Could you check a few things on this model? Use its own coordinates, in mm. Round coordinates to 2 decimals unless told otherwise and drop trailing zeros. Loops run counter-clockwise (first coordinate to the right, second up) from the corner with the lowest first, then second, coordinate; pieces in that order, holes last. Notation, with made-up numbers: (52.5, 56.25) -> (94.5, 56.25) arc R13 ccw to (94.5, 68.25) -> close; hole circle Ø11 at (16.5, 45.5). An arc over 180 degrees is marked (long way). Write each question's results on one line, items separated by ' | '.
from build123d import *

# Parameters (mm, degrees)
SKETCH1_W           = 70
SKETCH1_H           = 60
SKETCH1_R           = 2.125
SKETCH1_R_2         = 2.5
SKETCH1_R_3         = 1.5
SKETCH1_R_4         = 6
BOSS_EXTRUDE1_DEPTH = 6


with BuildPart() as part:
    # Sketch1 → Boss-Extrude1 (new body)
    with BuildSketch(Plane(origin=(0, 0, 0), x_dir=(1, 0, 0), z_dir=(0, 1, 0))):
        with Locations((0, -5)):
            Rectangle(SKETCH1_W, SKETCH1_H)
        with Locations((-9.450109616, -25)):
            Circle(SKETCH1_R, mode=Mode.SUBTRACT)
        with Locations((-17.450109616, -25)):
            Circle(SKETCH1_R, mode=Mode.SUBTRACT)
        with Locations((-25, -17.5)):
            Circle(SKETCH1_R_2, mode=Mode.SUBTRACT)
        with Locations((25, -17.5)):
            Circle(SKETCH1_R_2, mode=Mode.SUBTRACT)
        with Locations((-16.22, 0)):
            Circle(SKETCH1_R_3, mode=Mode.SUBTRACT)
        Circle(SKETCH1_R_4, mode=Mode.SUBTRACT)
        with Locations((-25, 17.5)):
            Circle(SKETCH1_R_2, mode=Mode.SUBTRACT)
        with Locations((16.22, 0)):
            Circle(SKETCH1_R_3, mode=Mode.SUBTRACT)
        with Locations((25, 17.5)):
            Circle(SKETCH1_R_2, mode=Mode.SUBTRACT)
    extrude(amount=BOSS_EXTRUDE1_DEPTH)


solid = part.part
1) I'm going to push a flat-ended pin straight in: pin 1 (10 mm diameter, centred on x = -26.5, z = -11, fed in from -Y). Where does the tip first touch, or does it pass through?
Model answer:
pin 1: stops at y = 0
2) I want a section at B-B, the plane x = -25. Write out the boundary of the cut face in (y, z), plus the area to 3 significant figures.
Model answer:
outline: (0, -25) -> (6, -25) -> (6, -20) -> (0, -20) -> close; (0, -15) -> (6, -15) -> (6, 15) -> (0, 15) -> close; (0, 20) -> (6, 20) -> (6, 35) -> (0, 35) -> close | area: 300 mm2
3) I want a section at C-C, the plane z = 0. Write out the boundary of the cut face in (x, y), plus the area to 3 significant figures.
Model answer:
outline: (-35, 0) -> (-17.72, 0) -> (-17.72, 6) -> (-35, 6) -> close; (-14.72, 0) -> (-6, 0) -> (-6, 6) -> (-14.72, 6) -> close; (6, 0) -> (14.72, 0) -> (14.72, 6) -> (6, 6) -> close; (17.72, 0) -> (35, 0) -> (35, 6) -> (17.72, 6) -> close | area: 312 mm2
4) I want a section at A-A, the plane z = 19. Write out the boundary of the cut face in (x, y).
Model answer:
outline: (-35, 0) -> (-27, 0) -> (-27, 6) -> (-35, 6) -> close; (-23, 0) -> (23, 0) -> (23, 6) -> (-23, 6) -> close; (27, 0) -> (35, 0) -> (35, 6) -> (27, 6) -> close
5) If we mould it in two halves opening along X, with no side actions, what happens to faces 1 (the flat face through (7, 6, 5)), 2 (the flat face through (-35, 3, 5)), 3 (the cylindrical face through (-6, 3, 0))? For each: released by +X, released by -X, zero draft, split by the parting line, or undercut.
Model answer:
face 1: zero draft | face 2: released by -X | face 3: undercut
6) I need wall thicknesses on line 1 (X direction, y = 1.65, z = 25); line 2 (X direction, y = 4.15, z = 17.5); line 3 (Z direction, x = -25, y = 4.4). Which ranges of each line are inside material? Lowest first, please.
Model answer:
line 1: x = -35 to -19.58, -15.33 to -11.58, -7.33 to 35 | line 2: x = -35 to -27.5, -22.5 to 22.5, 27.5 to 35 | line 3: z = -25 to -20, -15 to 15, 20 to 35
7) I want a section at D-D, the plane x = 0. Write out the boundary of the cut face in (y, z), plus the area to 3 significant figures.
Model answer:
outline: (0, -25) -> (6, -25) -> (6, -6) -> (0, -6) -> close; (0, 6) -> (6, 6) -> (6, 35) -> (0, 35) -> close | area: 288 mm2
